Geometry check sheet. Reference: the model listing, model coordinates, mm. Face numbers are marked on the shaded views. A direction names the side the tool comes from. Coordinates: 2 decimals unless noted, no trailing zeros. Loops run counter-clockwise (first coordinate to the right, second up) from the corner with the lowest first, then second, coordinate; pieces in that order, holes last. Notation, with made-up numbers: (20, -7.75) -> (78, -7.75) arc R12 ccw to (78, 14.25) -> close; hole circle Ø6 at (5.25, 1.5). An arc over 180 degrees is marked (long way). Answer as a JSON object with one key per item and string values.
from build123d import *

# Parameters (mm, degrees)
SKETCH1_R               = 20
BOSS_EXTRUDE1_DEPTH     = 120
CUT_EXTRUDE5_DEPTH      = 124.288280059
CUT_EXTRUDE5_DEPTH_BACK = 124.288280059
SKETCH2_W               = 17.5
SKETCH2_H               = 60
SKETCH2_W_2             = 24.890093951
CUT_EXTRUDE7_DEPTH      = 124.718430317
CUT_EXTRUDE7_DEPTH_BACK = 124.718430317
SKETCH6_R               = 3
FILLET1_R               = 3


with BuildPart() as part:
    # Sketch1 → Boss-Extrude1 (new, symmetric)
    with BuildSketch(Plane(origin=(0, 0, 0), x_dir=(1, 0, 0), z_dir=(0, 1, 0))):
        with Locations(Location((0, 0, 0), (0, 0, 270))):
            Circle(SKETCH1_R)
    extrude(amount=BOSS_EXTRUDE1_DEPTH, both=True)

    # Sketch2 → Cut-Extrude5 (cut, two sides: drawn at the far end of the back side and taken through both)
    with BuildSketch(Plane.XY.offset(-CUT_EXTRUDE5_DEPTH_BACK)):
        with Locations((-11.25, 0)):
            Rectangle(SKETCH2_W, SKETCH2_H)
        with Locations((14.945046976, 0)):
            Rectangle(SKETCH2_W_2, SKETCH2_H)
    extrude(amount=CUT_EXTRUDE5_DEPTH + CUT_EXTRUDE5_DEPTH_BACK, mode=Mode.SUBTRACT)

    # Sketch6 → Cut-Extrude7 (cut, two sides: drawn at the far end of the back side and taken through both)
    with BuildSketch(Plane(origin=(2.5, 0, 0), x_dir=(0, 0, -1), z_dir=(1, 0, 0)).offset(-CUT_EXTRUDE7_DEPTH_BACK)):
        Circle(SKETCH6_R)
    extrude(amount=CUT_EXTRUDE7_DEPTH + CUT_EXTRUDE7_DEPTH_BACK, mode=Mode.SUBTRACT)

    # Sketch7 → Cut-Revolve1 (revolve, cut)
    with BuildSketch(Plane(origin=(0, 0, 0), x_dir=(0, 0, -1), z_dir=(1, 0, 0))):
        with BuildLine():
            Line((-30, 104), (-10, 104))
            ThreePointArc((-10, 104), (-20, 94), (-30, 104))
        make_face()
    revolve(axis=Axis((0, 104, 30), (0, 0, -1)), mode=Mode.SUBTRACT)

    # Fillet1
    fillet1_edges = [part.edges().sort_by_distance(p)[0] for p in [
        (0, -120, -20),
        (0, 120, -20),
    ]]
    fillet(fillet1_edges, radius=FILLET1_R)


solid = part.part
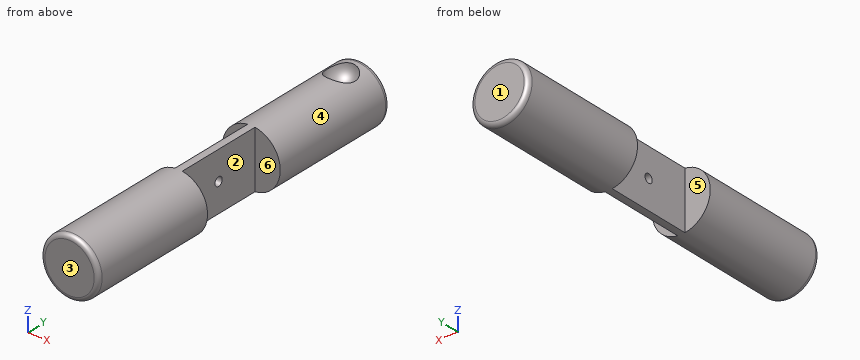
1. Thickness scan on probe 1 along Y at (x, z) = (0.4, 0); probe 2 along Y at (x, z) = (-7, -5.5); probe 3 along Z at (x, y) = (-0.8, 0). Record the ranges inside material, lowest first. Write a range as from..to.
Evaluation:
{"probe 1": "y = -120..-3, 3..120", "probe 2": "y = -120..-30, 30..120", "probe 3": "z = -19.98..-3, 3..19.98"}
2. Section check D-D, the plane y = -34. Record the boundary of the cut face in (x, z), then the cut area to 3 significant figures.
Evaluation:
{"outline": "circle Ø40 at (0, 0)", "area": "1,260 mm^2"}
3. Tool access check on the marked faces 4, 5 and 6. Record the directions out of +Z, -Z, +X, -X, +Y, -Y that give a thin tool (end or side, any length) a straight path to the whole face; none if there is none.
Evaluation:
{"face 4": "+Y, -Y", "face 5": "+Z, -Z, -X", "face 6": "+Z, -Z, +X"}
4. Section check A-A, the plane y = 0. Record the boundary of the cut face in (x, z).
Evaluation:
{"outline": "(-2.5, -19.84) arc R20 ccw to (2.5, -19.84) -> (2.5, -3) -> (-2.5, -3) -> close; (-2.5, 3) -> (2.5, 3) -> (2.5, 19.84) arc R20 ccw to (-2.5, 19.84) -> close"}
5. Section check C-C, the plane x = 0. Record the boundary of the cut face in (y, z), then the cut area to 3 significant figures.
Evaluation:
{"outline": "(-120, -17) arc R3 ccw to (-117, -20) -> (117, -20) arc R3 ccw to (120, -17) -> (120, 17) arc R3 ccw to (117, 20) -> (114, 20) arc R10 cw to (94, 20) -> (-117, 20) arc R3 ccw to (-120, 17) -> close; hole circle Ø6 at (0, 0)", "area": "9,410 mm^2"}
6. Section check B-B, the plane z = 0. Record the boundary of the cut face in (x, y), then the cut area to 3 significant figures.
Evaluation:
{"outline": "(-20, -117) arc R3 ccw to (-17, -120) -> (17, -120) arc R3 ccw to (20, -117) -> (20, -30) -> (2.5, -30) -> (2.5, -3) -> (-2.5, -3) -> (-2.5, -30) -> (-20, -30) -> close; (-20, 30) -> (-2.5, 30) -> (-2.5, 3) -> (2.5, 3) -> (2.5, 30) -> (20, 30) -> (20, 117) arc R3 ccw to (17, 120) -> (-17, 120) arc R3 ccw to (-20, 117) -> close", "area": "7,460 mm^2"}
7. Mould release check, pull along Y, two halves, no side actions. Record for the marked faces 1, 2 and 3: released by +Y, released by -Y, zero draft, split by the parting line, or undercut.
Evaluation:
{"face 1": "released by +Y", "face 2": "undercut", "face 3": "released by -Y"}
8. Depth check by flat-ended pin: P1, Ø12, axis at y = -73.5, z = 6, coming from the +X side; P2, Ø12, axis at y = -10, z = -1, coming from the -X side; P3, Ø1.5, axis at y = -28, z = -10.5, coming from the +X side. Enter the tip coordinate at first touch or a pass-through.
Evaluation:
{"P1": "stops at x = 20", "P2": "stops at x = -2.5", "P3": "stops at x = 2.5"}
